```python
from build123d import *

# Parameters (mm, degrees)
SKETCH1_R           = 2.1
BOSS_EXTRUDE1_DEPTH = 100


with BuildPart() as part:
    # Sketch1 → Boss-Extrude1 (new body, symmetric)
    with BuildSketch(Plane.XY):
        Polygon((5.499339828, 6.56), (3.59, 4.650660172), (-3.59, 4.650660172), (-5.499339828, 6.56), (-5.499339828, 8.2), (-3.1, 8.2), (-4.9, 10), (-10, 10), (-10, 4.9), (-8.2, 3.1), (-8.2, 5.499339828), (-6.56, 5.499339828), (-4.650660172, 3.59), (-4.650660172, -3.59), (-6.56, -5.499339828), (-8.2, -5.499339828), (-8.2, -3.1), (-10, -4.9), (-10, -10), (-4.9, -10), (-3.1, -8.2), (-5.499339828, -8.2), (-5.499339828, -6.56), (-3.59, -4.650660172), (3.59, -4.650660172), (5.499339828, -6.56), (5.499339828, -8.2), (3.1, -8.2), (4.9, -10), (10, -10), (10, -4.9), (8.2, -3.1), (8.2, -5.499339828), (6.56, -5.499339828), (4.650660172, -3.59), (4.650660172, 3.59), (6.56, 5.499339828), (8.2, 5.499339828), (8.2, 3.1), (10, 4.9), (10, 10), (4.9, 10), (3.1, 8.2), (5.499339828, 8.2), align=None)
        Circle(SKETCH1_R, mode=Mode.SUBTRACT)
    extrude(amount=BOSS_EXTRUDE1_DEPTH, both=True)


solid = part.part
```
Build history of the part. All positions in model axes, mm. A direction names the side the tool comes from. Round coordinates to 2 decimals unless told otherwise and drop trailing zeros. Order: outer loops, then holes, each group sorted by start corner. A loop starts at its lowest first (then second) coordinate and runs counter-clockwise, first axis right, second up. Notation, with made-up numbers: (-26, -36.5) - (-13, -36.5) arc R21 ccw to (-13, -16.5) - close; hole circle Ø2 at (-29, 30). An arc over 180 degrees is marked (long way). Use a Markdown table: item, result.
1) Flat gauge pins, fed straight in: pin 1 Ø3.5 at (y, z) = (1, -15.5) entering from -X; pin 2 Ø8 at (x, z) = (0, -33.5) entering from -Y; pin 3 Ø0.7 at (y, z) = (4.5, -0.5) entering from +X; pin 4 Ø3.5 at (x, y) = (0, 0) entering from -Z. Where does each tip first touch, or does it go through?
Recorded:
| item | result |
|---|---|
| pin 1 | stops at x = -4.65 |
| pin 2 | stops at y = -9.1 |
| pin 3 | stops at x = 9.95 |
| pin 4 | passes through |
2) Wall check: L1, parallel to X at y = 6, z = 56.5; L2, parallel to Y at x = 0, z = -38.5; L3, parallel to X at y = -7.5, z = 0.5. Give the ranges that are in metal, low to high.
Recorded:
| item | result |
|---|---|
| L1 | x = -10 to -4.94, 4.94 to 10 |
| L2 | y = -4.65 to -2.1, 2.1 to 4.65 |
| L3 | x = -10 to -5.5, 5.5 to 10 |
3) Tool access for faces 1 (the face through (-4.651, 0, 1)), 2 (the face through (-7, 10, 1)): list every direction of +Z, -Z, +X, -X, +Y, -Y with a clear straight run to the whole face (end or side of a thin tool).
Recorded:
| item | result |
|---|---|
| face 1 | +Z, -Z |
| face 2 | +Z, -Z, +X, -X, +Y |
4) Saw through at A-A on x = 0. Write the cut outline in (y, z), and give its area (3 significant figures).
Recorded:
| item | result |
|---|---|
| outline | (-4.65, -100) - (-2.1, -100) - (-2.1, 100) - (-4.65, 100) - close; (2.1, -100) - (4.65, -100) - (4.65, 100) - (2.1, 100) - close |
| area | 1,020 mm² |
5) Pull direction X, two halves, no side cores. Call faces 3 (the face through (-2.4, 0.1, 100)), 4 (the face through (-10, -7, 1)), 5 (the face through (0, -4.651, 1)): pulls with the +X half, pulls with the -X half, needs draft (parallel to the pull), parting line crosses it, or undercut.
Recorded:
| item | result |
|---|---|
| face 3 | needs draft |
| face 4 | pulls with the -X half |
| face 5 | undercut |
